```python
from build123d import *

# Parameters (mm, degrees)
BOSS_EXTRUDE2_DEPTH       = 88.9
SKETCH2_W                 = 25.4
SKETCH2_H                 = 108.331
BOSS_EXTRUDE3_DEPTH       = 136.652
M4X0_7_TAPPED_HOLE2_D     = 3.3
M4X0_7_TAPPED_HOLE2_DEPTH = 9.906
M4X0_7_TAPPED_HOLE2_TIP   = 0.991420021
SKETCH5_W                 = 44.196
SKETCH5_H                 = 44.196
BOSS_EXTRUDE4_DEPTH       = 9.144


with BuildPart() as part:
    # Sketch1 → Boss-Extrude2 (new body)
    with BuildSketch(Plane(origin=(0, 0, 0), x_dir=(1, 0, 0), z_dir=(0, 1, 0))):
        Polygon((-82.55, 86.075791262), (107.95, 86.075791262), (107.95, -66.324208738), (-82.55, -66.324208738), (-82.55, -187.355208738), (-107.95, -187.355208738), (-107.95, 86.075791262), align=None)
    extrude(amount=BOSS_EXTRUDE2_DEPTH)

    # Sketch2 → Boss-Extrude3 (add)
    with BuildSketch(Plane(origin=(0, 88.9, 0), x_dir=(1, 0, 0), z_dir=(0, 1, 0))):
        with Locations((-95.25, -133.189708738)):
            Rectangle(SKETCH2_W, SKETCH2_H)
    extrude(amount=BOSS_EXTRUDE3_DEPTH)

    # M4x0.7 Tapped Hole2
    with Locations(Plane(origin=(95.25, 0, -73.375791262), x_dir=(0, 0, -1), z_dir=(0, -1, 0))):
        with Locations((0, 0), (0, -192.024), (-127, -48.26), (-248.031, -192.024), (-165.1, -192.024)):
            Hole(M4X0_7_TAPPED_HOLE2_D / 2, depth=M4X0_7_TAPPED_HOLE2_DEPTH)
            with Locations((0, 0, -(M4X0_7_TAPPED_HOLE2_DEPTH + M4X0_7_TAPPED_HOLE2_TIP / 2))):  # 118° drill point
                Cone(0, M4X0_7_TAPPED_HOLE2_D / 2, M4X0_7_TAPPED_HOLE2_TIP, mode=Mode.SUBTRACT)

    # Sketch5 → Boss-Extrude4 (add)
    with BuildSketch(Plane.ZY.offset(107.95)):
        with Locations((-39.847791262, 66.802)):
            Rectangle(SKETCH5_W, SKETCH5_H)
    extrude(amount=BOSS_EXTRUDE4_DEPTH)


solid = part.part
```
Check sheet for the modelled part. Datum: model origin and axes. Units: mm. A direction names the side the tool comes from. Give positions to 0.01 mm unless a question says otherwise; leave off trailing zeros. Order: outer loops, then holes, each group sorted by start corner. A loop starts at its lowest first (then second) coordinate and runs counter-clockwise, first axis right, second up. Notation, with made-up numbers: M 54.25,-34.75 L 97.25,-34.75 A13 cw 97.25,-18.75 Z; hole C 23.25,62.5 d11. An arc over 180 degrees is marked long. Answer in a Markdown table with one row per item. Add a question column.
Q1. Access from +Z, -Z, +X, -X, +Y, -Y to the whole of each face (thin tool, end or side, straight path). Record for faces 4 (the flat face through (-112, 66, -17.75)), 5 (the flat face through (-3, 88.9, -5)), 6 (the flat face through (-112, 44.704, -40)).
Q2. Sectioned sample at D-D, the plane y = 17. Record the boundary of the cut face in (x, z), and give its area (3 significant figures).
Q3. Gauge pin test, flat ends, axial feed: pin 1 Ø4.5 at (x, y) = (-113, 75) entering from +Z; pin 2 Ø2 at (y, z) = (202.5, 145.5) entering from -X; pin 3 Ø10 at (x, y) = (-113, 71.5) entering from -Z. Record the tip position at first contact, or that the pin passes through.
Q4. Thickness scan on L1, parallel to Z at x = 95, y = 7; L2, parallel to Y at x = 5, z = -59; L3, parallel to Z at x = 76, y = 60. Record the ranges inside material, lowest first.
Q5. Release check for a two-part mould opening along Z. For faces 1 (the flat face through (-107.95, 86, 83)), 2 (the flat face through (-112, 66, -61.946)), 3 (the flat face through (14, 44, 66.324)) record: released by +Z, released by -Z, zero draft, split by the parting line, or undercut.
Q6. Sectioned sample at A-A, the plane y = 82. Record the boundary of the cut face in (x, z), and give its area (3 significant figures).
Q7. Sectioned sample at B-B, the plane z = 150. Record the boundary of the cut face in (x, y).
Q8. Sectioned sample at C-C, the plane x = 80.5. Record the boundary of the cut face in (y, z).
Verdict:
| question | item | result |
|---|---|---|
| 1 | face 4 | +Z, -X, +Y, -Y |
| 1 | face 5 | -Z, +X, -X, +Y |
| 1 | face 6 | +Z, -Z, -X, -Y |
| 2 | outline | M -107.95,-86.08 L 107.95,-86.08 L 107.95,66.32 L -82.55,66.32 L -82.55,187.36 L -107.95,187.36 Z |
| 2 | area | 36,000 mm² |
| 3 | pin 1 | z = -17.75 |
| 3 | pin 2 | x = -107.95 |
| 3 | pin 3 | z = -61.95 |
| 4 | L1 | -86.08 to -75.01, -71.74 to 66.32 |
| 4 | L2 | 0 to 88.9 |
| 4 | L3 | -86.08 to 66.32 |
| 5 | face 1 | zero draft |
| 5 | face 2 | released by -Z |
| 5 | face 3 | released by +Z |
| 6 | outline | M -117.09,-61.95 L -107.95,-61.95 L -107.95,-86.08 L 107.95,-86.08 L 107.95,66.32 L -82.55,66.32 L -82.55,187.36 L -107.95,187.36 L -107.95,-17.75 L -117.09,-17.75 Z |
| 6 | area | 36,400 mm² |
| 7 | outline | M -107.95,0 L -82.55,0 L -82.55,225.55 L -107.95,225.55 Z |
| 8 | outline | M 0,-86.08 L 88.9,-86.08 L 88.9,66.32 L 0,66.32 Z |
